Autodesk Inventor part; units mm, degrees
ref_plane "YZ Plane" through (0, 0, 0) normal (1, 0, 0) x (0, 1, 0)
ref_plane "XZ Plane" through (0, 0, 0) normal (0, 1, 0) x (-1, 0, 0)
ref_plane "XY Plane" through (0, 0, 0) normal (0, 0, 1) x (1, 0, 0)
sketch "Sketch1" plane through (0, 0, 0) normal (0, 0, 1) x (1, 0, 0)
  circle A0 centre (0, 0) radius 27.5
  line L0 (-27.5, 0) -> (27.5, 0)
  line L1 (27.5, 0) -> (27.5, -36)
  line L2 (27.5, -36) -> (-27.5, -36)
  line L3 (-27.5, -36) -> (-27.5, 0)
  line L4 (27.5, -30) -> (-27.5, -30)
  point P0 (20, 0)
  point P1 (20, 0)
  point P2 (20, 0)
  dimension "d0" = 55
  dimension "d1" = 36
  dimension "d2" = 6
  dimension "d7" = 20
extrude "Extrusion1" add sketch "Sketch1" along normal blind 6 contours L0 A0 | L1 L4 L3 A0 | A0 L0
extrude "Extrusion2" add sketch "Sketch1" along normal blind 100 contours L1 L2 L3 L4
sketch "Sketch2" plane through (0, 0, 6) normal (0, 0, 1) x (1, 0, 0)
  arc A0 (27.5, 0) -> (-27.5, 0) centre (0, 0) ccw
  line L0 (-27.5, -30) -> (-21.5, -30)
  line L1 (-21.5, -30) -> (-21.5, -20)
  line L2 (-21.5, -20) -> (-27.5, -20)
  line L3 (-27.5, -20) -> (-27.5, -30)
  point P0 (20, 0)
  point P1 (14.1421, 14.1421)
  point P2 (0, 20)
  point P3 (-14.1421, 14.1421)
  point P4 (-20, 0)
  point P5 (-14.1421, -14.1421)
  point P6 (0, -20)
  point P7 (14.1421, -14.1421)
  dimension "d8" = 20
  dimension "d11" = 360
  dimension "d20" = 6
  dimension "d21" = 10
hole "Hole1" at (20, 0, 6) at (0, 20, 6) at (-14.1421, 14.1421, 6) at (-20, 0, 6) at (-14.1421, -14.1421, 6) at (0, -20, 6) at (14.1421, -14.1421, 6) at (14.1421, 14.1421, 6) direction (0, 0, -1) diameter 6.6 end through all
extrude "Extrusion3" add sketch "Sketch2" along normal blind 10
mirror "Mirror3" about plane through (0, 0, 0) normal (1, 0, 0) of "Extrusion3"
chamfer "Chamfer1" distance 10 angle 45 2 edges at (-24.5, -20, 16) (24.5, -20, 16)
sketch "Sketch3" plane through (-27.5, -30, 100) normal (0, 1, 0) x (1, 0, 0)
  line L0 (55, 0) -> (0, 0)
  line L1 (55, 84) -> (55, 0)
  arc A0 (30.65, 55) -> (24.35, 55) centre (27.5, 55) ccw
  arc A1 (24.35, 15) -> (30.65, 15) centre (27.5, 15) ccw
  line L2 (30.65, 55) -> (30.65, 15)
  line L3 (24.35, 55) -> (24.35, 15)
  point P0 (27.5, 100)
  dimension "d27" = 15
  dimension "d28" = 40
  dimension "d29" = 3.15
  dimension "d30" = 3.15
extrude "Extrusion4" cut sketch "Sketch3" against normal through all
fillet "Fillet1" radius 10 2 edges at (27.5, -33, 100) (-27.5, -33, 100)
properties part number "c920_plate"
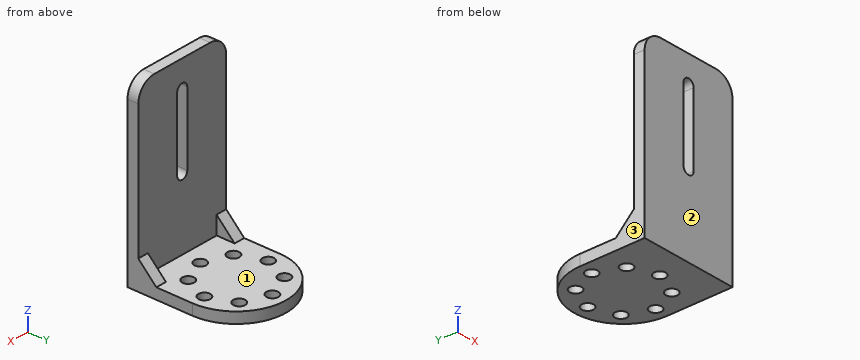
Could you check a few things on this model? Use its own coordinates, in mm. Face numbers are marked on the shaded views. Round coordinates to 2 decimals unless told otherwise and drop trailing zeros. Order: outer loops, then holes, each group sorted by start corner. A loop starts at its lowest first (then second) coordinate and runs counter-clockwise, first axis right, second up. Notation, with made-up numbers: M 55.5,-4.75 L 113.5,-4.75 A25 ccw 113.5,18.25 Z; hole C 27,27 d8. An arc over 180 degrees is marked long. One line per question, with ' | ' between items. Start each with the question number.
(1) Suppose I cut it at A-A on x = 0. List the corners of the cut face in (y, z) for me, then the cut area to 3 significant figures.
(2) Suppose I cut it at C-C on x = 20. List the corners of the cut face in (y, z) for me.
(3) Suppose I cut it at B-B on z = 81. List the corners of the cut face in (x, y) for me, then the cut area to 3 significant figures.
(4) Suppose I cut it at D-D on y = 20. List the corners of the cut face in (x, z) for me, then the cut area to 3 significant figures.
(5) For P1, Ø1, axis at x = 2.5, z = 34, coming from the +Y side; P2, Ø12, axis at x = -1, z = 68.5, coming from the -Y side; P3, Ø6, axis at x = 14.14, y = -14.14, coming from the -Z side; P4, Ø3, axis at x = 14, y = 1.5, coming from the +Z side, each with a flat end and sliding along its axis, tell me the tip position at first contact or that it passes through.
(6) Thinking about a two-plate mould opening in X: for the marked faces 1, 2 and 3, which applies, +X half, -X half, draft (parallel to the pull), parting line (faces both ways), or undercut?
(7) Please list where these lines run through material, in increasing order: line 1 along X through (y, z) = (0, 4.2); line 2 along Y through (x, z) = (0, 3.6); line 3 along X through (y, z) = (-20, 4).
Geometry results:
1) outline: M -36,0 L -23.3,0 L -23.3,6 L -30,6 L -30,41.85 L -36,41.85 Z; M -36,88.15 L -30,88.15 L -30,100 L -36,100 Z; M -16.7,0 L 16.7,0 L 16.7,6 L -16.7,6 Z; M 23.3,0 L 27.5,0 L 27.5,6 L 23.3,6 Z | area: 588 mm²
2) outline: M -36,0 L -3.3,0 L -3.3,6 L -30,6 L -30,99.68 L -36,99.68 Z; M 3.3,0 L 18.87,0 L 18.87,6 L 3.3,6 Z
3) outline: M -27.5,-36 L -3.15,-36 L -3.15,-30 L -27.5,-30 Z; M 3.15,-36 L 27.5,-36 L 27.5,-30 L 3.15,-30 Z | area: 292 mm²
4) outline: M -18.87,0 L -3.3,0 L -3.3,6 L -18.87,6 Z; M 3.3,0 L 18.87,0 L 18.87,6 L 3.3,6 Z | area: 187 mm²
5) P1: y = -30 | P2: y = -36 | P3: through | P4: z = 6
6) face 1: undercut | face 2: draft | face 3: -X half
7) line 1: -27.5 to -23.3, -16.7 to 16.7, 23.3 to 27.5 | line 2: -36 to -23.3, -16.7 to 16.7, 23.3 to 27.5 | line 3: -27.5 to -3.3, 3.3 to 27.5
